Solid Edge part; units mm, degrees
sketch "Sketch1" plane through (0, 0, 0) normal (0, 0, 1) x (1, 0, 0)
  line L0 (-19.25, -6.625) -> (19.25, -6.625)
  line L1 (19.25, -6.625) -> (19.25, 6.625)
  line L2 (19.25, 6.625) -> (-19.25, 6.625)
  line L3 (-19.25, 6.625) -> (-19.25, -6.625)
  dimension "D1" = 19.25
  dimension "D2" = 19.25
extrude "Protrusion1" add sketch "Sketch1" along normal blind 8.5
sketch "Sketch2" plane through (0, 0, 0) normal (0, 0, -1) x (1, 0, 0)
  circle A0 centre (-15, 0) radius 3.15
  circle A1 centre (15, 0) radius 3.15
extrude "Extrusionsausprägung_2" add sketch "Sketch2" along normal blind 5
fillet "Verrundung_1" radius 6.55 4 edges at (19.25, -6.625, 4.25) (19.25, 6.625, 4.25) (-19.25, -6.625, 4.25) (-19.25, 6.625, 4.25)
sketch "Sketch3" plane through (0, 0, 8.5) normal (0, 0, 1) x (1, 0, 0)
  circle A0 centre (0, 0) radius 5
extrude "Extrusionsausschnitt_2" cut sketch "Sketch3" against normal blind 199.2649
chamfer "Fase_2" distance 1 angle 45 16 edges at (0, 6.625, 8.5) (-17.3315, 4.7065, 8.5) (-19.25, 0, 8.5) (-17.3315, -4.7065, 8.5) (0, -6.625, 8.5) (17.3315, -4.7065, 8.5) (19.25, 0, 8.5) (0, -6.625, 0) (17.3315, -4.7065, 0) (19.25, 0, 0) (0, 6.625, 0) (-17.3315, 4.7065, 0) (-19.25, 0, 0) (-17.3315, -4.7065, 0) (-18.15, 0, -5) (11.85, 0, -5)
chamfer "Fase_3" distance 0.4 angle 45 2 edges at (-5, 0, 0) (-5, 0, 8.5)
Could you check a few things on this model? Use its own coordinates, in mm. A direction names the side the tool comes from. Round coordinates to 2 decimals unless told otherwise and drop trailing zeros. Loops run counter-clockwise (first coordinate to the right, second up) from the corner with the lowest first, then second, coordinate; pieces in that order, holes last. Notation, with made-up numbers: (-7, 19) - (49, 19) arc R16 cw to (49, 23) - close; hole circle Ø11 at (52.25, 48.5). An arc over 180 degrees is marked (long way). Answer as CSV lines item,"result".
1. Please list where these lines run through material, in increasing order: line 1 along Y through (x, z) = (0, 5.75) (3 decimals); line 2 along Z through (x, y) = (-10.5, 5); line 3 along X through (y, z) = (0, -4.5). Write a range as [from, to].
Filled in:
line 1,"y = [-6.625, -5], [5, 6.625]"
line 2,"z = [0, 8.5]"
line 3,"x = [-17.65, -12.35], [12.35, 17.65]"
2. On a 3-axis mill with a long thin cutter (end or side, diameter ignored), from which of +Z, -Z, +X, -X, +Y, -Y can I reach the whole of each face in a straight line? I mean faces 1 (the face through (-18.147, 0.138, -1.972)), 2 (the face through (-1.08, -4.88, 4.3)). Say none if no direction works.
Filled in:
face 1,"-Z"
face 2,"+Z, -Z"
3. For pin 1 Ø2 at (y, z) = (5, 1) entering from -X; pin 2 Ø1 at (x, y) = (-7.5, 1.5) entering from -Z, each with a flat end and sliding along its axis, tell me the tip position at first contact or that it passes through.
Filled in:
pin 1,"stops at x = -17.94"
pin 2,"stops at z = 0"
4. We'd pull the mould along X, two halves only. Please class faces 3 (the face through (-4, -4, 0)), 4 (the face through (-16.791, -4.077, 0.174)), 5 (the face through (16.791, 4.077, 0.174)): +X half, -X half, draft (parallel to the pull), parting line (faces both ways), or undercut.
Filled in:
face 3,"undercut"
face 4,"-X half"
face 5,"+X half"
5. I want a section at C-C on z = -2.5. List the corners of the cut face in (x, y) for me, then the cut area to 3 significant figures.
Filled in:
outline,"circle Ø6.3 at (-15, 0); circle Ø6.3 at (15, 0)"
area,"62.3 mm^2"
6. I want a section at A-A on x = 0. List the corners of the cut face in (y, z) for me (3 decimals), then the cut area to 3 significant figures.
Filled in:
outline,"(-6.625, 1) - (-5.625, 0) - (-5.4, 0) - (-5, 0.4) - (-5, 8.1) - (-5.4, 8.5) - (-5.625, 8.5) - (-6.625, 7.5) - close; (5, 0.4) - (5.4, 0) - (5.625, 0) - (6.625, 1) - (6.625, 7.5) - (5.625, 8.5) - (5.4, 8.5) - (5, 8.1) - close"
area,"25.3 mm^2"
7. I want a section at B-B on z = 1.75. List the corners of the cut face in (x, y) for me (3 decimals), then the cut area to 3 significant figures.
Filled in:
outline,"(-19.25, -0.075) arc R6.55 ccw to (-12.7, -6.625) - (12.7, -6.625) arc R6.55 ccw to (19.25, -0.075) - (19.25, 0.075) arc R6.55 ccw to (12.7, 6.625) - (-12.7, 6.625) arc R6.55 ccw to (-19.25, 0.075) - close; hole circle Ø10 at (0, 0)"
area,"395 mm^2"
